Model file for the job. Use its own axes, mm. Give positions to 0.01 mm unless a question says otherwise; leave off trailing zeros. Write each loop counter-clockwise with the first axis right and the second up, starting at its lowest first coordinate (ties: lowest second). Pieces come first, ordered by that corner, then holes. Notation, with made-up numbers: (-31.5, 34.5) - (0.5, 34.5) arc R21 ccw to (0.5, 71.5) - close; hole circle Ø2 at (-3, 51.5). An arc over 180 degrees is marked (long way). One line per item, written item: value. Start each with the question number.
(1) Cut at D-D, the plane z = -4.25. List the corners of the cut face in (x, y), and give its area (3 significant figures).
(2) Mould opens along Z. For faces 1 (the face through (-14, -6, -23.685)), 2 (the face through (-18.08, -6.26, -10.78)), 3 (the face through (-38.723, -6, -17)) say: pulls with the +Z half, pulls with the -Z half, needs draft (parallel to the pull), parting line crosses it, or undercut.
(3) Cut at A-A, the plane y = -8.25. List the corners of the cut face in (x, z) (1 decimal), and give its area (3 significant figures).
(4) Probe L1, parallel to Z at x = -13, y = -7; L2, parallel to X at y = -1.25, z = -8; L3, parallel to X at y = -0.75, z = -6.75. List the from-to ranges inside material, lowest first.
(5) Cut at B-B, the plane x = -15. List the corners of the cut face in (y, z).
(6) Cut at C-C, the plane z = -10.25. List the corners of the cut face in (x, y), and give its area (3 significant figures).
from build123d import *

# Parameters (mm, degrees)
F0_R     = 4.7625
F1_DEPTH = 12.7


with BuildPart() as f1:
    # F0 (on Front) → F1 (new body)
    with BuildSketch(Plane.XZ):
        Polygon((-38.722962, -10.984917), (-38.722962, -23.684917), (12.077038, -23.684917), (12.077038, -10.984917), (-6.972962, -10.984917), (-6.972962, 1.715083), (-19.672962, 1.715083), (-19.672962, -10.984917), align=None)
        with Locations((-13.322962, -10.984917)):
            Circle(F0_R, mode=Mode.SUBTRACT)
        Polygon((-19.672962, 1.715083), (-38.722962, -10.984917), (-19.672962, -10.984917), align=None)
        Polygon((-6.972962, -10.984917), (12.077038, -10.984917), (-6.972962, 1.715083), align=None)
    extrude(amount=F1_DEPTH)


solid = f1.part
Answers follow:
1. outline: (-28.62, -12.7) - (1.97, -12.7) - (1.97, 0) - (-28.62, 0) - close
1. area: 389 mm²
2. face 1: pulls with the -Z half
2. face 2: undercut
2. face 3: needs draft
3. outline: (-38.7, -23.7) - (12.1, -23.7) - (12.1, -11) - (-7, 1.7) - (-19.7, 1.7) - (-38.7, -11) - close; hole circle Ø9.5 at (-13.3, -11)
3. area: 977 mm²
4. L1: z = -23.68 to -15.74, -6.23 to 1.72
4. L2: x = -34.25 to -17.03, -9.61 to 7.6
4. L3: x = -32.37 to -15.5, -11.14 to 5.72
5. outline: (-12.7, -23.68) - (0, -23.68) - (0, -15.44) - (-12.7, -15.44) - close; (-12.7, -6.53) - (0, -6.53) - (0, 1.72) - (-12.7, 1.72) - close
6. outline: (-37.62, -12.7) - (-18.03, -12.7) - (-18.03, 0) - (-37.62, 0) - close; (-8.62, -12.7) - (10.97, -12.7) - (10.97, 0) - (-8.62, 0) - close
6. area: 498 mm²
